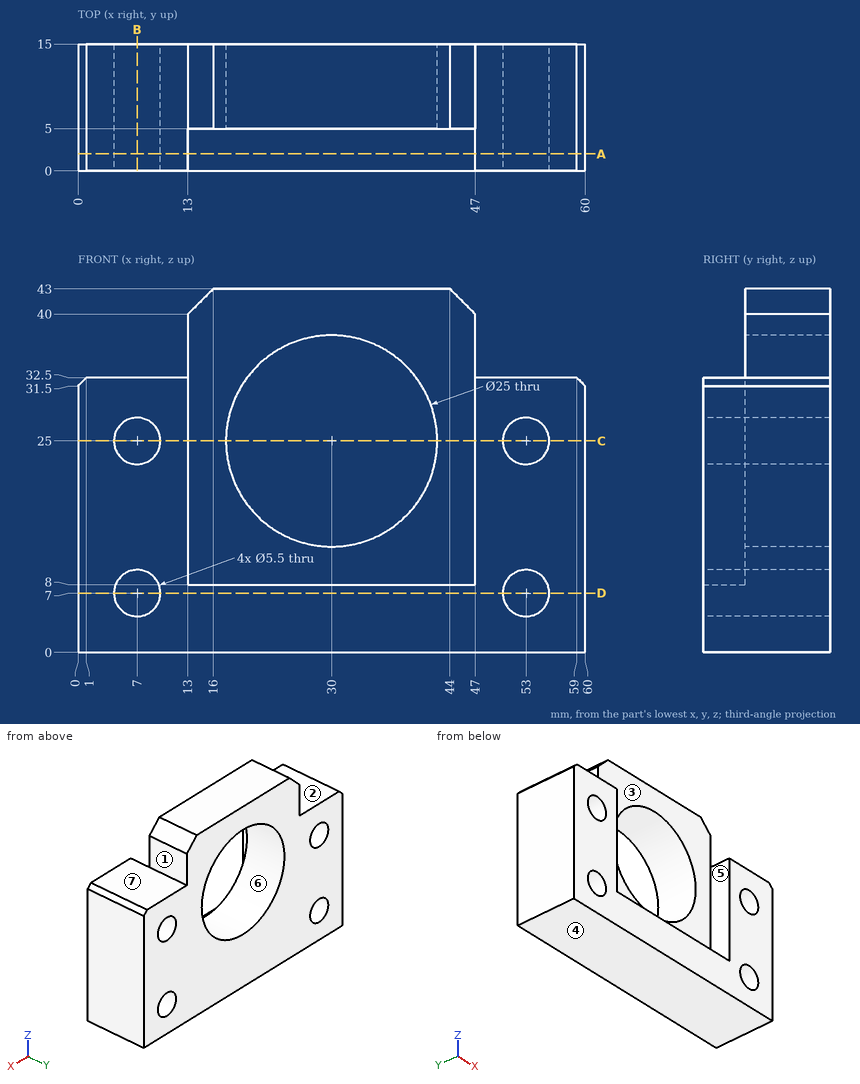
Here's the drawing with two shaded views (mm, measured from the low corner). I have some questions. A direction names the side the tool comes from. Give positions to 0.01 mm unless a question says otherwise; leave off trailing zeros. Loops run counter-clockwise (first coordinate to the right, second up) from the corner with the lowest first, then second, coordinate; pieces in that order, holes last. Notation, with made-up numbers: M 2,54 L 25,54 A26 cw 25,76 Z; hole C 74,72 d2. An arc over 180 degrees is marked long. One line per item, written item: value.
1) On a 3-axis mill with a long thin cutter (end or side, diameter ignored), from which of +Z, -Z, +X, -X, +Y, -Y can I reach the whole of each face in a straight line? I mean the marked faces 1, 2 and 3. Say none if no direction works.
Geometry check:
face 1: +Z, +X, +Y, -Y
face 2: +Z, -X, +Y, -Y
face 3: +Z, -Y
2) Please list where these lines run through material, in increasing order: line 1 (Z direction, x = 7, y = 11.75); line 2 (Z direction, x = 5.5, y = 4); line 3 (Z direction, x = 30, y = 7).
Geometry check:
line 1: z = 0 to 4.25, 9.75 to 22.25, 27.75 to 32.5
line 2: z = 0 to 4.7, 9.3 to 22.7, 27.3 to 32.5
line 3: z = 0 to 12.5, 37.5 to 43
3) I'm going to push flat-ended pins straight in: pin 1 (8 mm diameter, centred on y = 12, z = 37, fed in from +X); pin 2 (4 mm diameter, centred on x = 32, y = 2.5, fed in from +Z); pin 3 (6 mm diameter, centred on x = 9, y = 10, fed in from +Z). Where does each tip first touch, or does it pass through?
Geometry check:
pin 1: stops at x = 47
pin 2: stops at z = 8
pin 3: stops at z = 32.5
4) Thinking about a two-plate mould opening in Z: for the marked faces 4, 5, 6 and 7, which applies, +Z half, -Z half, draft (parallel to the pull), parting line (faces both ways), or undercut?
Geometry check:
face 4: -Z half
face 5: draft
face 6: undercut
face 7: +Z half
5) Imagine slicing it at C-C on z = 25. Write out the boundary of the cut face in (x, y).
Geometry check:
outline: M 0,0 L 4.25,0 L 4.25,15 L 0,15 Z; M 9.75,0 L 13,0 L 13,5 L 17.5,5 L 17.5,15 L 9.75,15 Z; M 42.5,5 L 47,5 L 47,0 L 50.25,0 L 50.25,15 L 42.5,15 Z; M 55.75,0 L 60,0 L 60,15 L 55.75,15 Z
6) Imagine slicing it at D-D on z = 7. Write out the boundary of the cut face in (x, y), and give its area (3 significant figures).
Geometry check:
outline: M 0,0 L 4.25,0 L 4.25,15 L 0,15 Z; M 9.75,0 L 50.25,0 L 50.25,15 L 9.75,15 Z; M 55.75,0 L 60,0 L 60,15 L 55.75,15 Z
area: 735 mm²
7) Imagine slicing it at B-B on x = 7. Write out the boundary of the cut face in (y, z), and give its area (4 significant figures).
Geometry check:
outline: M 0,0 L 15,0 L 15,4.25 L 0,4.25 Z; M 0,9.75 L 15,9.75 L 15,22.25 L 0,22.25 Z; M 0,27.75 L 15,27.75 L 15,32.5 L 0,32.5 Z
area: 322.5 mm²
8) Imagine slicing it at A-A on y = 2. Write out the boundary of the cut face in (x, z), and give its area (3 significant figures).
Geometry check:
outline: M 0,0 L 60,0 L 60,31.5 L 59,32.5 L 47,32.5 L 47,8 L 13,8 L 13,32.5 L 1,32.5 L 0,31.5 Z; hole C 7,7 d5.5; hole C 7,25 d5.5; hole C 53,7 d5.5; hole C 53,25 d5.5
area: 1,020 mm²
